Verification items for the finished model (mm, model axes). A direction names the side the tool comes from. Coordinates: 2 decimals unless noted, no trailing zeros. Write each loop counter-clockwise with the first axis right and the second up, starting at its lowest first coordinate (ties: lowest second). Pieces come first, ordered by that corner, then holes. Notation, with made-up numbers: M -30,27 L -23,27 A31 ccw -23,57 Z; hole C -17.75,77 d1. An arc over 180 degrees is marked long. One line per item, written item: value.
```python
from build123d import *

# Parameters (mm, degrees)
F0_W     = 50
F0_H     = 55
F1_DEPTH = 50
F2_W     = 40
F2_H     = 45
F3_DEPTH = 45
F4_W     = 40
F4_H     = 40
F5_DEPTH = 5


with BuildPart() as f1:
    # F0 (on Top) → F1 (new body)
    with BuildSketch(Plane.XY):
        Rectangle(F0_W, F0_H)
    extrude(amount=F1_DEPTH)

    # F2 (on face) → F3 (cut)
    with BuildSketch(Plane.XY.offset(50)):
        Rectangle(F2_W, F2_H)
    extrude(amount=-F3_DEPTH, mode=Mode.SUBTRACT)

    # F4 (on face) → F5 (cut)
    with BuildSketch(Plane.XZ.offset(27.5)):
        with Locations((0, 30)):
            Rectangle(F4_W, F4_H)
    extrude(amount=-F5_DEPTH, mode=Mode.SUBTRACT)


solid = f1.part
```
Item 1: Cross-section at A-A, the plane z = 8. Enter the section's corners in (x, y).
The answers:
outline: M -25,-27.5 L 25,-27.5 L 25,27.5 L -25,27.5 Z; hole M -20,-22.5 L 20,-22.5 L 20,22.5 L -20,22.5 Z
Item 2: Go/stop test with flat-tipped pins: P1, Ø4, axis at x = -9, z = 43.5, coming from the -Y side; P2, Ø1.5, axis at x = 4, y = -24, coming from the +Z side; P3, Ø1, axis at x = -1.5, y = -7.5, coming from the +Z side. Record where each tip stops, or that it passes through.
The answers:
P1: stops at y = 22.5
P2: stops at z = 10
P3: stops at z = 5
Item 3: Scan lines: line 1 (X direction, y = 0.5, z = 14); line 2 (Y direction, x = 7, z = 6); line 3 (Z direction, x = -9, y = -4). Record each from-to range of solid material in increasing order.
The answers:
line 1: x = -25 to -20, 20 to 25
line 2: y = -27.5 to -22.5, 22.5 to 27.5
line 3: z = 0 to 5
Item 4: Draft check along X on faces 3 (the face through (25, 0, 25)), 4 (the face through (0, -25, 10)), 5 (the face through (-25, 0, 25)), 6 (the face through (0, 0, 5)). Enter one of: released by +X, released by -X, zero draft, split by the parting line, or undercut.
The answers:
face 3: released by +X
face 4: undercut
face 5: released by -X
face 6: undercut
Item 5: Cross-section at C-C, the plane z = 28. Enter the section's corners in (x, y).
The answers:
outline: M -25,-27.5 L -20,-27.5 L -20,22.5 L 20,22.5 L 20,-27.5 L 25,-27.5 L 25,27.5 L -25,27.5 Z
Item 6: Access from +Z, -Z, +X, -X, +Y, -Y to the whole of each face (thin tool, end or side, straight path). Record for faces 1 (the face through (0, -22.5, 8)), 2 (the face through (-2, 23, 50)).
The answers:
face 1: +Z
face 2: +Z, +X, -X, +Y, -Y
Item 7: Cross-section at B-B, the plane y = -1. Enter the section's corners in (x, z).
The answers:
outline: M -25,0 L 25,0 L 25,50 L 20,50 L 20,5 L -20,5 L -20,50 L -25,50 Z
